Autodesk Inventor part; units mm, degrees
ref_plane "YZ Plane" through (0, 0, 0) normal (1, 0, 0) x (0, 1, 0)
ref_plane "XZ Plane" through (0, 0, 0) normal (0, 1, 0) x (-1, 0, 0)
ref_plane "XY Plane" through (0, 0, 0) normal (0, 0, 1) x (1, 0, 0)
sketch "Sketch1" plane through (0, 0, 0) normal (0, 1, 0) x (-1, 0, 0)
  circle A0 centre (0, 0) radius 55
  line L0 (480, 1020) -> (-520, 1020)
  line L1 (-520, 1020) -> (-520, -515)
  line L2 (-520, -515) -> (480, -515)
  line L3 (480, -515) -> (480, 1020)
  line L4 (267, -266) -> (-327, -266) construction
  circle A1 centre (132, -175) radius 15
  circle A2 centre (-97, -255) radius 15
  circle A3 centre (-8, -360) radius 20
  circle A4 centre (-15, 765) radius 55
  dimension "d0" = 110
  dimension "d1" = 515
  dimension "d2" = 1020
  dimension "d3" = 520
  dimension "d4" = 480
  dimension "d5" = 30
  dimension "d6" = 30
  dimension "d7" = 40
  dimension "d8" = 155
  dimension "d9" = 255
  dimension "d10" = 340
  dimension "d11" = 110
  dimension "d13" = 505
  dimension "d14" = 765
extrude "Extrusion1" add sketch "Sketch1" along normal blind 150
properties part number "protoPlinth"
Part model, mm, in its own coordinate system. Round coordinates to 2 decimals unless told otherwise and drop trailing zeros. Write each loop counter-clockwise with the first axis right and the second up, starting at its lowest first coordinate (ties: lowest second). Pieces come first, ordered by that corner, then holes. Notation, with made-up numbers: M -39,-11.75 L 11,-11.75 A10 ccw 11,-6.75 Z; hole C 64.25,31.5 d6. An arc over 180 degrees is marked long. Return JSON: item names as keys, results as strings. Group by question number.
(1) Pin check, flat tip, straight feed: pin 1 Ø12 at (x, z) = (181.5, 641) entering from -Y. Stop position of the tip, or through.
(2) Two-plate mould, pull along Z, no slides. Class faces 1 (the face through (-480, 74, 242)), 2 (the face through (13, 74, 1020)), 3 (the face through (88.94, 73.95, -267.65)): +Z half, -Z half, draft (parallel to the pull), parting line (faces both ways), or undercut.
(3) Drill centre lines: probe 1 along Z at (x, y) = (97, 45); probe 2 along Z at (x, y) = (8, 37); probe 3 along Z at (x, y) = (98.5, 17). Where is each one in solid material? Low to high.
(4) Saw through at A-A on z = -255. Write the cut outline in (x, y).
(5) Saw through at B-B on x = 97. Write the cut outline in (y, z).
Returned:
{
 "1": {"pin 1": "y = 0"},
 "2": {"face 1": "draft", "face 2": "+Z half", "face 3": "undercut"},
 "3": {"probe 1": "-515 to -270, -240 to 1020", "probe 2": "-515 to -380, -340 to -54.42, 54.42 to 710.45, 819.55 to 1020", "probe 3": "-515 to -269.92, -240.08 to 1020"},
 "4": {"outline": "M -480,0 L 82,0 L 82,150 L -480,150 Z; M 112,0 L 520,0 L 520,150 L 112,150 Z"},
 "5": {"outline": "M 0,-515 L 150,-515 L 150,-270 L 0,-270 Z; M 0,-240 L 150,-240 L 150,1020 L 0,1020 Z"}
}
